Design review of the part built by this model. Coordinates are the model's own, in mm. Coordinates: 2 decimals unless noted, no trailing zeros. Loops run counter-clockwise (first coordinate to the right, second up) from the corner with the lowest first, then second, coordinate; pieces in that order, holes last. Notation, with made-up numbers: (61.25, 83.25) - (80.25, 83.25) arc R28 ccw to (80.25, 118.25) - close; hole circle Ø8 at (-9, -21.5). An arc over 180 degrees is marked (long way). Return JSON: item names as keys, results as strings. Group by question number.
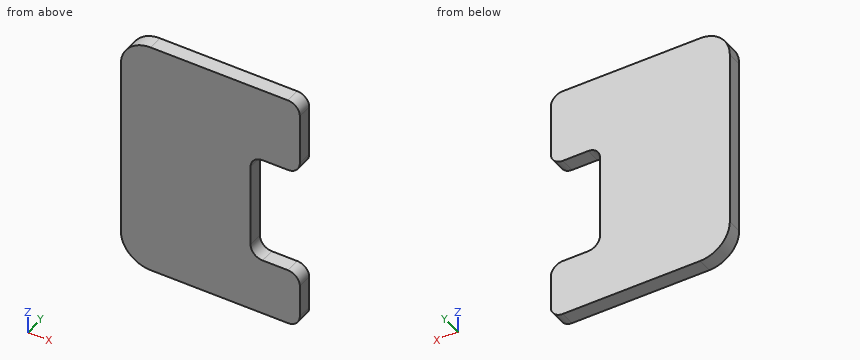
from build123d import *

# Parameters (mm, degrees)
SKETCH1_W           = 38.1
SKETCH1_H           = 50.8
BOSS_EXTRUDE1_DEPTH = 3.175
SKETCH2_W           = 10.4775
SKETCH2_H           = 22.86
CUT_EXTRUDE2_DEPTH  = 32.908355097
FILLET1_R           = 2.54
FILLET2_R           = 6.35


with BuildPart() as part:
    # Sketch1 → Boss-Extrude1 (new body)
    with BuildSketch(Plane(origin=(0, 0, 0), x_dir=(1, 0, 0), z_dir=(0, 1, 0))):
        Rectangle(SKETCH1_W, SKETCH1_H)
    extrude(amount=BOSS_EXTRUDE1_DEPTH)

    # Sketch2 → Cut-Extrude2 (cut, through all)
    with BuildSketch(Plane(origin=(0, 3.175, 0), x_dir=(1, 0, 0), z_dir=(0, 1, 0))):
        with Locations((13.81125, 1.905)):
            Rectangle(SKETCH2_W, SKETCH2_H)
    extrude(amount=-CUT_EXTRUDE2_DEPTH, mode=Mode.SUBTRACT)

    # Fillet1
    fillet1_edges = [part.edges().sort_by_distance(p)[0] for p in [
        (19.05, 1.5875, -13.335),
        (19.05, 1.5875, 9.525),
        (8.5725, 1.5875, 9.525),
        (8.5725, 1.5875, -13.335),
        (19.05, 1.5875, 25.4),
        (19.05, 1.5875, -25.4),
    ]]
    fillet(fillet1_edges, radius=FILLET1_R)

    # Fillet2
    fillet2_edges = [part.edges().sort_by_distance(p)[0] for p in [
        (-19.05, 1.5875, 25.4),
        (-19.05, 1.5875, -25.4),
    ]]
    fillet(fillet2_edges, radius=FILLET2_R)


solid = part.part
Item 1: Add section D-D (x = 9.5). State the section outline as (y, z) points (1 decimal), then the cut area to 3 significant figures.
Item 2: For P1, Ø1.6, axis at y = 1.5, z = -4.5, coming from the +X side; P2, Ø6, axis at x = 11, z = 3, coming from the -Y side, all flat-tipped, find the tip position at first contact; note any pin that passes through.
Item 3: Add section A-A (x = 15). State the section outline as (y, z) points (3 decimals), then the cut area to 3 significant figures.
Item 4: To check wall thickness, follow line 1 (Z direction, x = 9.5, y = 0.95); line 2 (Z direction, x = 12, y = 1.6) (3 decimals); line 3 (X direction, y = 2.55, z = -6.5). State the ranges of each line that lie inside material, in increasing order. Write a range as from..to.
Answers below:
{
 "1": {"outline": "(0, -25.4) - (3.2, -25.4) - (3.2, -12.8) - (0, -12.8) - close; (0, 8.9) - (3.2, 8.9) - (3.2, 25.4) - (0, 25.4) - close", "area": "92.4 mm^2"},
 "2": {"P1": "stops at x = 8.57", "P2": "stops at y = 0"},
 "3": {"outline": "(0, -25.4) - (3.175, -25.4) - (3.175, -13.335) - (0, -13.335) - close; (0, 9.525) - (3.175, 9.525) - (3.175, 25.4) - (0, 25.4) - close", "area": "88.7 mm^2"},
 "4": {"line 1": "z = -25.4..-12.76, 8.95..25.4", "line 2": "z = -25.4..-13.335, 9.525..25.4", "line 3": "x = -19.05..8.57"}
}
